```python
from build123d import *

# Parameters (mm, degrees)
F0_R     = 88.9
F0_R_2   = 63.5
F1_DEPTH = 939.8
F2_R     = 69.0499
F2_R_2   = 63.5
F3_DEPTH = 76.2
F4_R     = 69.05625
F5_DEPTH = 76.2
F6_SIZE  = 1.524


with BuildPart() as f1:
    # F0 (on Right) → F1 (new body, symmetric)
    with BuildSketch(Plane.YZ):
        Circle(F0_R)
        Circle(F0_R_2, mode=Mode.SUBTRACT)
    extrude(amount=F1_DEPTH, both=True)

    # F2 (on face) → F3 (cut)
    with BuildSketch(Plane.YZ.offset(939.8)):
        Circle(F2_R)
        Circle(F2_R_2, mode=Mode.SUBTRACT)
    extrude(amount=-F3_DEPTH, mode=Mode.SUBTRACT)

    # F4 (on face) → F5 (cut)
    with BuildSketch(Plane(origin=(-939.8, 0, 0), x_dir=(0, -1, 0), z_dir=(-1, 0, 0))):
        Circle(F4_R)
    extrude(amount=-F5_DEPTH, mode=Mode.SUBTRACT)

    # F6
    f6_edges = [f1.edges().sort_by_distance(p)[0] for p in [
        (-939.8, -88.9, 0),
        (939.8, -88.9, 0),
    ]]
    chamfer(f6_edges, length=F6_SIZE)


solid = f1.part
```
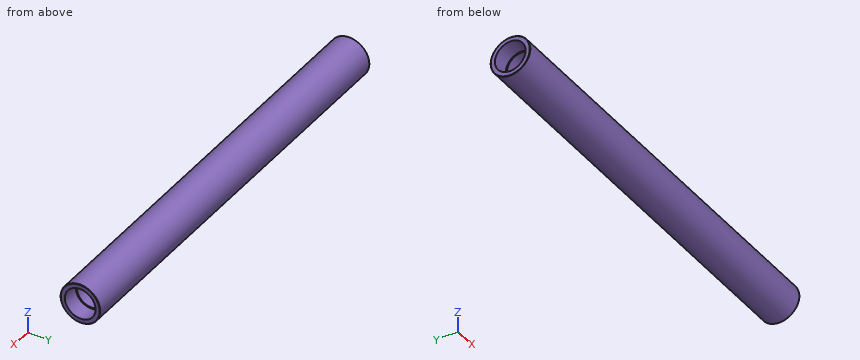
Source: CAD feature listing. Evaluate the final solid. Frame: model axes, mm. Coordinates: 2 decimals unless noted, no trailing zeros. Order: outer loops, then holes, each group sorted by start corner. A loop starts at its lowest first (then second) coordinate and runs counter-clockwise, first axis right, second up. Notation, with made-up numbers: (7.25, 37) - (23.25, 37) arc R21 cw to (23.25, 59) - close; hole circle Ø9 at (-24, 5). An arc over 180 degrees is marked (long way). One line per item, written item: value.
1) Ray query, line 1 (Z direction, x = -176, y = -5); line 2 (Z direction, x = -888, y = 0); line 3 (Y direction, x = -434.5, z = 3). Return the intervals inside material, ascending. Write a range as [from, to].
Computed values:
line 1: z = [-88.76, -63.3], [63.3, 88.76]
line 2: z = [-88.9, -69.06], [69.06, 88.9]
line 3: y = [-88.85, -63.43], [63.43, 88.85]
2) Contact query for flat-ended pins moving along their axis: pin 1 (1 mm diameter, centred on x = -345, y = 64, fed in from +Z); pin 2 (1 mm diameter, centred on y = -26, z = -58.5, fed in from -X); pin 3 (1 mm diameter, centred on x = -327, y = 9, fed in from -Z). Output: stop coordinate, or through.
Computed values:
pin 1: stops at z = 62.22
pin 2: stops at x = -863.6
pin 3: stops at z = -88.49
3) Cut plane C-C on x = 678. Output: boundary loops of the cut face in (y, z), plus the area to 3 significant figures.
Computed values:
outline: circle Ø177.8 at (0, 0); hole circle Ø127 at (0, 0)
area: 12,200 mm^2
4) Cut plane A-A on z = 0. Output: boundary loops of the cut face in (x, y).
Computed values:
outline: (-939.8, -87.38) - (-938.28, -88.9) - (938.28, -88.9) - (939.8, -87.38) - (939.8, -69.05) - (863.6, -69.05) - (863.6, -63.5) - (-863.6, -63.5) - (-863.6, -69.06) - (-939.8, -69.06) - close; (-939.8, 69.06) - (-863.6, 69.06) - (-863.6, 63.5) - (863.6, 63.5) - (863.6, 69.05) - (939.8, 69.05) - (939.8, 87.38) - (938.28, 88.9) - (-938.28, 88.9) - (-939.8, 87.38) - close
